Geometry check sheet. Reference: the model listing, model coordinates, mm. Give positions to 0.01 mm unless a question says otherwise; leave off trailing zeros. Order: outer loops, then holes, each group sorted by start corner. A loop starts at its lowest first (then second) coordinate and runs counter-clockwise, first axis right, second up. Notation, with made-up numbers: M 78,71.25 L 132,71.25 A5 cw 132,77.25 Z; hole C 9.5,52 d2. An arc over 180 degrees is marked long. Put each result on its own line as item: value. Start each with the question number.
Q1. Material ranges on L1, parallel to Y at x = 0, z = 1; L2, parallel to X at y = -72, z = 1; L3, parallel to X at y = 33.5, z = 1.35, recorded low to high.
Q2. Go/stop test with a flat-tipped pin: pin 1 (2 mm diameter, centred on x = -22.22, y = -125.41, fed in from -Z). Record where the tip stops, or that it passes through.
Q3. Section check A-A on y = 29.5. Record the cut outline in (x, z) (3 decimals), then the cut area to 3 significant figures.
Q4. Section check B-B on z = 2.45. State how many separate pieces and enclosed holes the cut face has, then the cut area to 3 significant figures.
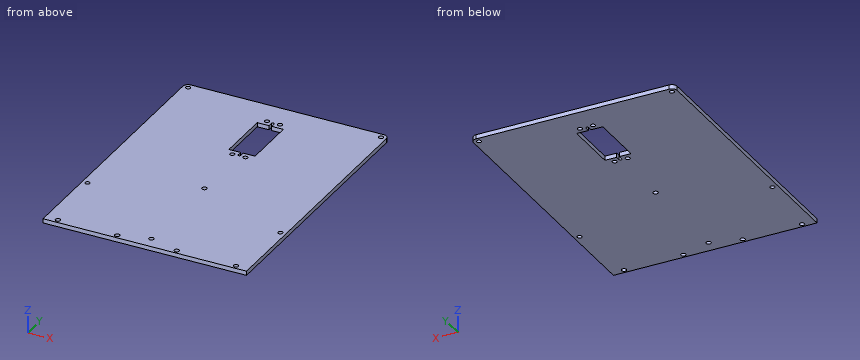
```python
from build123d import *

# Parameters (mm, degrees)
F0_W     = 152.4
F0_H     = 204.7875
F0_R     = 1.8288
F0_R_2   = 1.7272
F1_DEPTH = 3.175
F2_R     = 3.96875


with BuildPart() as f1:
    # F0 (on Top) → F1 (new body)
    with BuildSketch(Plane.XY):
        with Locations((0, -26.19375)):
            Rectangle(F0_W, F0_H)
        with Locations((-66.675, -125.4125)):
            Circle(F0_R, mode=Mode.SUBTRACT)
        with Locations((-22.225, -125.4125)):
            Circle(F0_R, mode=Mode.SUBTRACT)
        with Locations((-72.23125, -72.23125)):
            Circle(F0_R_2, mode=Mode.SUBTRACT)
        with Locations((0, -119.0625)):
            Circle(F0_R, mode=Mode.SUBTRACT)
        with Locations((22.225, -125.4125)):
            Circle(F0_R, mode=Mode.SUBTRACT)
        with Locations((66.675, -125.4125)):
            Circle(F0_R, mode=Mode.SUBTRACT)
        with Locations((0, -42.8625)):
            Circle(F0_R, mode=Mode.SUBTRACT)
        with Locations((72.23125, -72.23125)):
            Circle(F0_R_2, mode=Mode.SUBTRACT)
        with Locations((-4.8895, 6.528203)):
            Circle(F0_R_2, mode=Mode.SUBTRACT)
        with Locations((-72.23125, 72.23125)):
            Circle(F0_R_2, mode=Mode.SUBTRACT)
        with Locations((-4.8895, 56.312203)):
            Circle(F0_R_2, mode=Mode.SUBTRACT)
        with Locations((4.8895, 6.528203)):
            Circle(F0_R_2, mode=Mode.SUBTRACT)
        with BuildLine():
            Line((1.016, 55.169203), (1.016, 51.740203))
            Line((1.016, 51.740203), (9.779, 51.740203))
            Line((9.779, 51.740203), (9.779, 11.100203))
            Line((9.779, 11.100203), (1.016, 11.100203))
            Line((1.016, 11.100203), (1.016, 7.671203))
            ThreePointArc((1.016, 7.671203), (0, 6.655203), (-1.016, 7.671203))
            Line((-1.016, 7.671203), (-1.016, 11.100203))
            Line((-1.016, 11.100203), (-9.779, 11.100203))
            Line((-9.779, 11.100203), (-9.779, 51.740203))
            Line((-9.779, 51.740203), (-1.016, 51.740203))
            Line((-1.016, 51.740203), (-1.016, 55.169203))
            ThreePointArc((-1.016, 55.169203), (0, 56.185203), (1.016, 55.169203))
        make_face(mode=Mode.SUBTRACT)
        with Locations((4.8895, 56.312203)):
            Circle(F0_R_2, mode=Mode.SUBTRACT)
        with Locations((72.23125, 72.23125)):
            Circle(F0_R_2, mode=Mode.SUBTRACT)
    extrude(amount=F1_DEPTH)

    # F2
    f2_edges = [f1.edges().sort_by_distance(p)[0] for p in [
        (-76.2, 76.2, 1.5875),
        (76.2, 76.2, 1.5875),
    ]]
    fillet(f2_edges, radius=F2_R)


solid = f1.part
```
Results found:
1. L1: y = -128.59 to -120.89, -117.23 to -44.69, -41.03 to 6.66, 56.19 to 76.2
1. L2: x = -76.2 to -73.94, -70.52 to 70.52, 73.94 to 76.2
1. L3: x = -76.2 to -9.78, 9.78 to 76.2
2. pin 1: passes through
3. outline: M -76.2,0 L -9.779,0 L -9.779,3.175 L -76.2,3.175 Z; M 9.779,0 L 76.2,0 L 76.2,3.175 L 9.779,3.175 Z
3. area: 422 mm^2
4. separate pieces: 1
4. enclosed holes: 15
4. area: 30,300 mm^2
